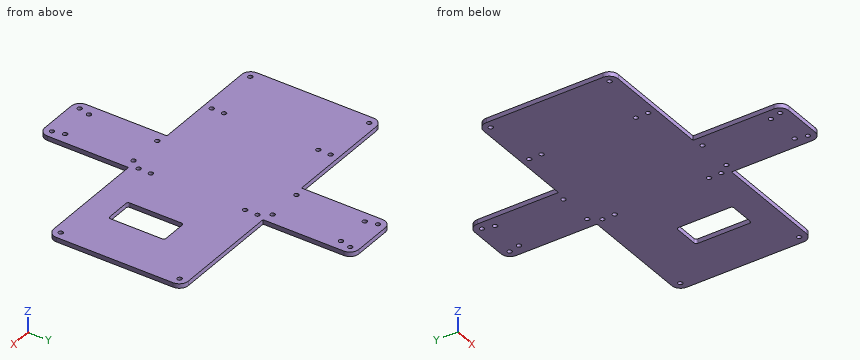
```python
from build123d import *

# Parameters (mm, degrees)
SKETCH_2_W      = 25
SKETCH_2_H      = 50
SKETCH_2_R      = 2
EXTRUDE_1_DEPTH = 4
FILLET_1_R      = 8
FILLET_2_R      = 2


with BuildPart() as part:
    # 草图2 → 凸台-拉伸1 (new body)
    with BuildSketch(Plane.XY):
        Polygon((-39.472146663, 69.287551935), (-144.472146663, 69.287551935), (-144.472146663, -50.712448065), (-39.472146663, -50.712448065), (-39.472146663, -130.712448065), (10.527853337, -130.712448065), (10.527853337, -50.712448065), (115.527853337, -50.712448065), (115.527853337, 69.287551935), (10.527853337, 69.287551935), (10.527853337, 149.287551935), (-39.472146663, 149.287551935), align=None)
        with Locations((60.527853337, -0.712448065)):
            Rectangle(SKETCH_2_W, SKETCH_2_H, mode=Mode.SUBTRACT)
        with Locations((-87.472146663, -43.712448065)):
            Circle(SKETCH_2_R, mode=Mode.SUBTRACT)
        with Locations((-87.472146663, -32.712448065)):
            Circle(SKETCH_2_R, mode=Mode.SUBTRACT)
        with Locations((7.527853337, -32.712448065)):
            Circle(SKETCH_2_R, mode=Mode.SUBTRACT)
        with Locations((7.527853337, -43.712448065)):
            Circle(SKETCH_2_R, mode=Mode.SUBTRACT)
        with Locations((7.527853337, 51.287551935)):
            Circle(SKETCH_2_R, mode=Mode.SUBTRACT)
        with Locations((7.527853337, 62.287551935)):
            Circle(SKETCH_2_R, mode=Mode.SUBTRACT)
        with Locations((-87.472146663, 51.287551935)):
            Circle(SKETCH_2_R, mode=Mode.SUBTRACT)
        with Locations((-87.472146663, 62.287551935)):
            Circle(SKETCH_2_R, mode=Mode.SUBTRACT)
        with Locations((-137.472146663, 62.287551935)):
            Circle(SKETCH_2_R, mode=Mode.SUBTRACT)
        with Locations((-137.472146663, -43.712448065)):
            Circle(SKETCH_2_R, mode=Mode.SUBTRACT)
        with Locations((-29.972146663, 132.287551935)):
            Circle(SKETCH_2_R, mode=Mode.SUBTRACT)
        with Locations((1.027853337, 132.287551935)):
            Circle(SKETCH_2_R, mode=Mode.SUBTRACT)
        with Locations((1.027853337, 71.287551935)):
            Circle(SKETCH_2_R, mode=Mode.SUBTRACT)
        with Locations((-29.972146663, 71.287551935)):
            Circle(SKETCH_2_R, mode=Mode.SUBTRACT)
        with Locations((3.527853337, 142.287551935)):
            Circle(SKETCH_2_R, mode=Mode.SUBTRACT)
        with Locations((-32.472146663, 142.287551935)):
            Circle(SKETCH_2_R, mode=Mode.SUBTRACT)
        with Locations((108.527853337, 62.287551935)):
            Circle(SKETCH_2_R, mode=Mode.SUBTRACT)
        with Locations((108.527853337, -43.712448065)):
            Circle(SKETCH_2_R, mode=Mode.SUBTRACT)
        with Locations((1.027853337, -52.712448065)):
            Circle(SKETCH_2_R, mode=Mode.SUBTRACT)
        with Locations((3.527853337, -123.712448065)):
            Circle(SKETCH_2_R, mode=Mode.SUBTRACT)
        with Locations((-32.472146663, -123.712448065)):
            Circle(SKETCH_2_R, mode=Mode.SUBTRACT)
        with Locations((-29.972146663, -113.712448065)):
            Circle(SKETCH_2_R, mode=Mode.SUBTRACT)
        with Locations((-29.972146663, -52.712448065)):
            Circle(SKETCH_2_R, mode=Mode.SUBTRACT)
        with Locations((1.027853337, -113.712448065)):
            Circle(SKETCH_2_R, mode=Mode.SUBTRACT)
    extrude(amount=EXTRUDE_1_DEPTH)

    # 圆角1
    fillet_1_edges = [part.edges().sort_by_distance(p)[0] for p in [
        (10.527853337, -130.712448065, 2),
        (-39.472146663, -130.712448065, 2),
        (-144.472146663, -50.712448065, 2),
        (-144.472146663, 69.287551935, 2),
        (-39.472146663, 149.287551935, 2),
        (10.527853337, 149.287551935, 2),
        (115.527853337, 69.287551935, 2),
        (115.527853337, -50.712448065, 2),
    ]]
    fillet(fillet_1_edges, radius=FILLET_1_R)

    # 圆角2
    fillet_2_edges = [part.edges().sort_by_distance(p)[0] for p in [
        (73.027853337, -25.712448065, 2),
        (73.027853337, 24.287551935, 2),
        (48.027853337, 24.287551935, 2),
        (48.027853337, -25.712448065, 2),
    ]]
    fillet(fillet_2_edges, radius=FILLET_2_R)


solid = part.part
```
For this review, take the finished solid that the model builds, in its own axes (mm). Coordinates: 2 decimals unless noted, no trailing zeros. Order: outer loops, then holes, each group sorted by start corner. A loop starts at its lowest first (then second) coordinate and runs counter-clockwise, first axis right, second up. Notation, with made-up numbers: (86, -21.5) - (119, -21.5) arc R28 cw to (119, 3.5) - close; hole circle Ø11 at (61, 89.25). An arc over 180 degrees is marked (long way). Answer as a JSON object with one key per item and string values. Group by question number.
1. For probe 1 along X at (y, z) = (-18, 1.4); probe 2 along Y at (x, z) = (64, 0.2); probe 3 along X at (y, z) = (-32, 3.85), list the stretches that pass through material, from the lowest coordinate up.
2. Clearance check with a flat-ended pin moving along its axis: P1, Ø1.2, axis at x = 43, z = 2.5, coming from the +Y side. State where the tip first meets the part, or that it passes through.
3. We need section B-B on x = 57. State the section outline as (y, z) points, then the cut area to 3 significant figures.
4. We need section D-D on y = -85.5. State the section outline as (x, z) points.
5. We need section A-A on y = 0. State the section outline as (x, z) points.
6. We need section C-C on x = -52. State the section outline as (y, z) points.
Final values:
{
 "1": {"probe 1": "-144.47 to 48.03, 73.03 to 115.53", "probe 2": "-50.71 to -25.71, 24.29 to 69.29", "probe 3": "-144.47 to -89.34, -85.6 to 5.66, 9.4 to 115.53"},
 "2": {"P1": "y = 69.29"},
 "3": {"outline": "(-50.71, 0) - (-25.71, 0) - (-25.71, 4) - (-50.71, 4) - close; (24.29, 0) - (69.29, 0) - (69.29, 4) - (24.29, 4) - close", "area": "280 mm²"},
 "4": {"outline": "(-39.47, 0) - (10.53, 0) - (10.53, 4) - (-39.47, 4) - close"},
 "5": {"outline": "(-144.47, 0) - (48.03, 0) - (48.03, 4) - (-144.47, 4) - close; (73.03, 0) - (115.53, 0) - (115.53, 4) - (73.03, 4) - close"},
 "6": {"outline": "(-50.71, 0) - (69.29, 0) - (69.29, 4) - (-50.71, 4) - close"}
}
